```python
from build123d import *

# Parameters (mm, degrees)
SKETCH1_W           = 38.1
SKETCH1_H           = 17.78
BOSS_EXTRUDE1_DEPTH = 9.525
SKETCH2_R           = 1.905
CUT_EXTRUDE1_DEPTH  = 12.7


with BuildPart() as part:
    # Sketch1 → Boss-Extrude1 (new, symmetric)
    with BuildSketch(Plane(origin=(0, 0, 0), x_dir=(1, 0, 0), z_dir=(0, 1, 0))):
        with Locations((19.05, 8.89)):
            Rectangle(SKETCH1_W, SKETCH1_H)
    extrude(amount=BOSS_EXTRUDE1_DEPTH, both=True)

    # Sketch2 → Cut-Extrude1 (cut)
    with BuildSketch(Plane(origin=(0, 9.525, 0), x_dir=(1, 0, 0), z_dir=(0, 1, 0))):
        with Locations(Location((31.75, 8.89, 0), (0, 0, 270))):
            Circle(SKETCH2_R)
        with Locations(Location((19.098327334, 9.996877933, 0), (0, 0, 270))):
            Circle(SKETCH2_R)
        with Locations(Location((12.7, 8.89, 0), (0, 0, 270))):
            Circle(SKETCH2_R)
        with Locations(Location((25.496470768, 7.787334072, 0), (0, 0, 270))):
            Circle(SKETCH2_R)
        with Locations(Location((13.188250266, 4.604682415, 0), (0, 0, 270))):
            Circle(SKETCH2_R)
    extrude(amount=-CUT_EXTRUDE1_DEPTH, mode=Mode.SUBTRACT)


solid = part.part
```
For this review, take the finished solid that the model builds, in its own axes (mm). A direction names the side the tool comes from. Coordinates: 2 decimals unless noted, no trailing zeros. Order: outer loops, then holes, each group sorted by start corner. A loop starts at its lowest first (then second) coordinate and runs counter-clockwise, first axis right, second up. Notation, with made-up numbers: (-10.75, 73) - (4.25, 73) arc R17 ccw to (4.25, 79) - close; hole circle Ø10 at (-20, 74.5). An arc over 180 degrees is marked (long way). Answer as a JSON object with one key per item and string values. Group by question number.
1. For probe 1 along X at (y, z) = (4.75, -8.75); probe 2 along X at (y, z) = (5.5, -10.5); probe 3 along X at (y, z) = (0, -8.89) (3 decimals), list the stretches that pass through material, from the lowest coordinate up.
2. We need section B-B on x = 31.75. State the section outline as (y, z) points (3 decimals), then the cut area to 3 significant figures.
3. Clearance check with a flat-ended pin moving along its axis: P1, Ø1.1, axis at x = 14, z = -4, coming from the +Y side (3 decimals). State where the tip first meets the part, or that it passes through.
4. We need section A-A on y = -1.5. State the section outline as (x, z) points (3 decimals), then the cut area to 3 significant figures.
5. For faces 5 (the flat face through (19, 9.525, -7)), 6 (the cylindrical face through (20.386, 3.264, -11.401)), list the 3-axis set-ups (+Z, -Z, +X, -X, +Y, -Y) from which the entire face can be reached by the end or side of a thin tool; tool diameter is ignored.
6. The part is to be moulded in two halves that separate along Z. For faces 1 (the flat face through (19, -9.525, -9)), 2 (the flat face through (19, 0, -17.78)), 3 (the cylindrical face through (11.97, 3.26, -7.13)), 4 (the flat face through (19, 0, 0)), say which applies: pulls with the +Z half, pulls with the -Z half, needs draft (parallel to the pull), parting line crosses it, or undercut.
7. We need section D-D on z = -4.5. State the section outline as (x, y) points (3 decimals), then the cut area to 3 significant figures.
8. We need section C-C on z = -8.89. State the section outline as (x, y) points (3 decimals), then the cut area to 3 significant figures.
Final values:
{
 "1": {"probe 1": "0 to 10.8, 14.6 to 17.66, 20.54 to 23.85, 27.14 to 29.85, 33.65 to 38.1", "probe 2": "0 to 11.68, 13.72 to 17.26, 20.94 to 30.73, 32.77 to 38.1", "probe 3": "0 to 10.795, 14.605 to 17.548, 20.649 to 23.943, 27.05 to 29.845, 33.655 to 38.1"},
 "2": {"outline": "(-9.525, -17.78) - (9.525, -17.78) - (9.525, -10.795) - (-3.175, -10.795) - (-3.175, -6.985) - (9.525, -6.985) - (9.525, 0) - (-9.525, 0) - close", "area": "290 mm²"},
 "3": {"P1": "y = -3.175"},
 "4": {"outline": "(0, -17.78) - (38.1, -17.78) - (38.1, 0) - (0, 0) - close; hole circle Ø3.81 at (12.7, -8.89); hole circle Ø3.81 at (13.188, -4.605); hole circle Ø3.81 at (19.098, -9.997); hole circle Ø3.81 at (25.496, -7.787); hole circle Ø3.81 at (31.75, -8.89)", "area": "620 mm²"},
 "5": {"face 5": "+Z, -Z, +X, -X, +Y", "face 6": "+Y"},
 "6": {"face 1": "needs draft", "face 2": "pulls with the -Z half", "face 3": "undercut", "face 4": "pulls with the +Z half"},
 "7": {"outline": "(0, -9.525) - (38.1, -9.525) - (38.1, 9.525) - (15.09, 9.525) - (15.09, -3.175) - (11.286, -3.175) - (11.286, 9.525) - (0, 9.525) - close", "area": "677 mm²"},
 "8": {"outline": "(0, -9.525) - (38.1, -9.525) - (38.1, 9.525) - (33.655, 9.525) - (33.655, -3.175) - (29.845, -3.175) - (29.845, 9.525) - (27.05, 9.525) - (27.05, -3.175) - (23.943, -3.175) - (23.943, 9.525) - (20.649, 9.525) - (20.649, -3.175) - (17.548, -3.175) - (17.548, 9.525) - (14.605, 9.525) - (14.605, -3.175) - (10.795, -3.175) - (10.795, 9.525) - (0, 9.525) - close", "area": "550 mm²"}
}
